Geometry: final body of the model. Coordinates: model frame, mm. Give positions to 0.01 mm unless a question says otherwise; leave off trailing zeros. Order: outer loops, then holes, each group sorted by start corner. A loop starts at its lowest first (then second) coordinate and runs counter-clockwise, first axis right, second up. Notation, with made-up numbers: M -19,36 L 16,36 A13 ccw 16,51 Z; hole C -1.5,31 d11. An arc over 180 degrees is marked long. Use CSV: the item, a comma, the result in double quotes.
```python
from build123d import *

# Parameters (mm, degrees)
SKETCH1_W           = 370
SKETCH1_H           = 169.75
BOSS_EXTRUDE1_DEPTH = 3
SKETCH3_W           = 20.2
SKETCH3_H           = 20.2
CUT_EXTRUDE1_DEPTH  = 4
SKETCH4_W           = 3.1
SKETCH4_H           = 55.5
SKETCH4_H_2         = 14.05
CUT_EXTRUDE2_DEPTH  = 4
FILLET1_R           = 10


with BuildPart() as part:
    # Sketch1 → Boss-Extrude1 (new body)
    with BuildSketch(Plane.XY):
        with Locations((440, -20.125)):
            Rectangle(SKETCH1_W, SKETCH1_H)
        with BuildLine():
            Line((427.05, 52.5), (427.05, 32.5))
            ThreePointArc((427.05, 32.5), (425, 30.45), (422.95, 32.5))
            Line((422.95, 32.5), (422.95, 52.5))
            ThreePointArc((422.95, 52.5), (425, 54.55), (427.05, 52.5))
        make_face(mode=Mode.SUBTRACT)
        with BuildLine():
            Line((572.95, 52.5), (572.95, 32.5))
            ThreePointArc((572.95, 32.5), (575, 30.45), (577.05, 32.5))
            Line((577.05, 32.5), (577.05, 52.5))
            ThreePointArc((577.05, 52.5), (575, 54.55), (572.95, 52.5))
        make_face(mode=Mode.SUBTRACT)
        with BuildLine():
            Line((427.05, -75), (427.05, -95))
            ThreePointArc((427.05, -95), (425, -97.05), (422.95, -95))
            Line((422.95, -95), (422.95, -75))
            ThreePointArc((422.95, -75), (425, -72.95), (427.05, -75))
        make_face(mode=Mode.SUBTRACT)
        with BuildLine():
            Line((572.95, -75), (572.95, -95))
            ThreePointArc((572.95, -95), (575, -97.05), (577.05, -95))
            Line((577.05, -95), (577.05, -75))
            ThreePointArc((577.05, -75), (575, -72.95), (572.95, -75))
        make_face(mode=Mode.SUBTRACT)
    extrude(amount=BOSS_EXTRUDE1_DEPTH)

    # Sketch3 → Cut-Extrude1 (cut, through all)
    with BuildSketch(Plane.XY.offset(3)):
        with Locations((279.9, -40.85)):
            Rectangle(SKETCH3_W, SKETCH3_H)
        with Locations((600.1, -40.85)):
            Rectangle(SKETCH3_W, SKETCH3_H)
    extrude(amount=-CUT_EXTRUDE1_DEPTH, mode=Mode.SUBTRACT)

    # Sketch4 → Cut-Extrude2 (cut, through all)
    with BuildSketch(Plane.XY.offset(3)):
        with Locations((268.4, 17)):
            Rectangle(SKETCH4_W, SKETCH4_H)
        with Locations((268.4, -77.975)):
            Rectangle(SKETCH4_W, SKETCH4_H_2)
        with Locations((611.6, -77.975)):
            Rectangle(SKETCH4_W, SKETCH4_H_2)
        with Locations((611.6, 17)):
            Rectangle(SKETCH4_W, SKETCH4_H)
    extrude(amount=-CUT_EXTRUDE2_DEPTH, mode=Mode.SUBTRACT)

    # Fillet1
    fillet1_edges = [part.edges().sort_by_distance(p)[0] for p in [
        (625, -105, 1.5),
        (255, -105, 1.5),
        (255, 64.75, 1.5),
        (625, 64.75, 1.5),
    ]]
    fillet(fillet1_edges, radius=FILLET1_R)


solid = part.part
```
1. Section B-B, the plane z = 2.2. Give the number of separate pieces and of enclosed holes in the cut face, plus the area to 3 significant figures.
Answer:
separate pieces,"1"
enclosed holes,"10"
area,"61,100 mm2"
2. Line query: line 1 (X direction, y = -75.5, z = 0.7); line 2 (X direction, y = 19.5, z = 2.6); line 3 (X direction, y = -45, z = 2.85). Output: solid intervals per line, ascending.
Answer:
line 1,"255 to 266.85, 269.95 to 422.95, 427.05 to 572.95, 577.05 to 610.05, 613.15 to 625"
line 2,"255 to 266.85, 269.95 to 610.05, 613.15 to 625"
line 3,"255 to 269.8, 290 to 590, 610.2 to 625"
3. Section A-A, the plane y = -0.5. Return the cut outline in (x, z), plus the area to 3 significant figures.
Answer:
outline,"M 255,0 L 266.85,0 L 266.85,3 L 255,3 Z; M 269.95,0 L 610.05,0 L 610.05,3 L 269.95,3 Z; M 613.15,0 L 625,0 L 625,3 L 613.15,3 Z"
area,"1,090 mm2"
